```python
from build123d import *

# Parameters (mm, degrees)
F0_W     = 32
F0_H     = 36.5
F0_W_2   = 28
F0_H_2   = 32.5
F1_DEPTH = 9
F0_R     = 0.9
F2_DEPTH = 2
F3_DEPTH = 5
F4_W     = 28
F4_H     = 2
F5_DEPTH = 2
F6_W     = 20
F6_H     = 7
F7_DEPTH = 2
F8_W     = 29
F8_H     = 27.5
F9_DEPTH = 5
F11_D    = 2.4
F13_D    = 2.4


with BuildPart() as f1:
    # F0 (on Top) → F1 (new body)
    with BuildSketch(Plane.XY):
        with Locations((-98.1993639427, 45.2269401511)):
            Rectangle(F0_W, F0_H)
        with Locations((-98.1993639427, 45.2269401511)):
            Rectangle(F0_W_2, F0_H_2, mode=Mode.SUBTRACT)
    extrude(amount=F1_DEPTH)

    # F0 (on Top) → F2 (join)
    with BuildSketch(Plane.XY):
        with Locations((-98.1993639427, 45.2269401511)):
            Rectangle(F0_W_2, F0_H_2)
        with Locations((-108.1993639427, 32.9769401511)):
            Circle(F0_R, mode=Mode.SUBTRACT)
        with Locations((-88.1993639427, 32.9769401511)):
            Circle(F0_R, mode=Mode.SUBTRACT)
        with Locations((-108.1993639427, 45.4769401511)):
            Circle(F0_R, mode=Mode.SUBTRACT)
        with Locations((-88.1993639427, 45.4769401511)):
            Circle(F0_R, mode=Mode.SUBTRACT)
    extrude(amount=F2_DEPTH)

    # F0 (on Top) → F3 (join)
    with BuildSketch(Plane.XY):
        with Locations((-108.1993639427, 32.9769401511)):
            Circle(F0_R)
        with Locations((-108.1993639427, 45.4769401511)):
            Circle(F0_R)
        with Locations((-88.1993639427, 32.9769401511)):
            Circle(F0_R)
        with Locations((-88.1993639427, 45.4769401511)):
            Circle(F0_R)
    extrude(amount=F3_DEPTH)

    # F4 (on face) → F5 (cut, through all)
    with BuildSketch(Plane.XZ.offset(-26.9769401511)):
        with Locations((-98.1993639427, 6)):
            Rectangle(F4_W, F4_H)
    extrude(amount=-F5_DEPTH, mode=Mode.SUBTRACT)

    # F6 (on face) → F7 (cut, through all)
    with BuildSketch(Plane(origin=(0, 63.4769401511, 0), x_dir=(-1, 0, 0), z_dir=(0, 1, 0))):
        with Locations((98.1993639427, 5.5)):
            Rectangle(F6_W, F6_H)
    extrude(amount=-F7_DEPTH, mode=Mode.SUBTRACT)

    # F8 (on face) → F9 (join)
    with BuildSketch(Plane(origin=(0, 0, 0), x_dir=(1, 0, 0), z_dir=(0, 0, -1))):
        with Locations((-98.1993639427, -46.4769401511)):
            Rectangle(F8_W, F8_H)
        with BuildLine():
            ThreePointArc((-99.1993639427, -35.7269401511), (-98.1993639427, -34.7269401511), (-97.1993639427, -35.7269401511))
            Line((-97.1993639427, -35.7269401511), (-86.6993639427, -35.7269401511))
            Line((-86.6993639427, -35.7269401511), (-86.6993639427, -45.4769401511))
            ThreePointArc((-86.6993639427, -45.4769401511), (-85.9922571615, -45.7698333699), (-85.6993639427, -46.4769401511))
            ThreePointArc((-85.6993639427, -46.4769401511), (-85.9922571615, -47.1840469322), (-86.6993639427, -47.4769401511))
            Line((-86.6993639427, -47.4769401511), (-86.6993639427, -57.2269401511))
            Line((-86.6993639427, -57.2269401511), (-97.1993639427, -57.2269401511))
            ThreePointArc((-97.1993639427, -57.2269401511), (-98.1993639427, -58.2269401511), (-99.1993639427, -57.2269401511))
            Line((-99.1993639427, -57.2269401511), (-109.6993639427, -57.2269401511))
            Line((-109.6993639427, -57.2269401511), (-109.6993639427, -47.4769401511))
            ThreePointArc((-109.6993639427, -47.4769401511), (-110.6993639427, -46.4769401511), (-109.6993639427, -45.4769401511))
            Line((-109.6993639427, -45.4769401511), (-109.6993639427, -35.7269401511))
            Line((-109.6993639427, -35.7269401511), (-99.1993639427, -35.7269401511))
        make_face(mode=Mode.SUBTRACT)
        with BuildLine():
            Line((-86.6993639427, -47.4769401511), (-86.6993639427, -45.4769401511))
            ThreePointArc((-86.6993639427, -45.4769401511), (-87.6993639427, -46.4769401511), (-86.6993639427, -47.4769401511))
        make_face()
        with BuildLine():
            ThreePointArc((-85.6993639427, -46.4769401511), (-85.9922571615, -45.7698333699), (-86.6993639427, -45.4769401511))
            Line((-86.6993639427, -45.4769401511), (-86.6993639427, -47.4769401511))
            ThreePointArc((-86.6993639427, -47.4769401511), (-85.9922571615, -47.1840469322), (-85.6993639427, -46.4769401511))
        make_face()
        with BuildLine():
            Line((-99.1993639427, -35.7269401511), (-97.1993639427, -35.7269401511))
            ThreePointArc((-97.1993639427, -35.7269401511), (-98.1993639427, -34.7269401511), (-99.1993639427, -35.7269401511))
        make_face()
        with BuildLine():
            ThreePointArc((-99.1993639427, -35.7269401511), (-98.1993639427, -36.7269401511), (-97.1993639427, -35.7269401511))
            Line((-97.1993639427, -35.7269401511), (-99.1993639427, -35.7269401511))
        make_face()
        with BuildLine():
            ThreePointArc((-108.6993639427, -46.4769401511), (-108.9922571615, -45.7698333699), (-109.6993639427, -45.4769401511))
            Line((-109.6993639427, -45.4769401511), (-109.6993639427, -47.4769401511))
            ThreePointArc((-109.6993639427, -47.4769401511), (-108.9922571615, -47.1840469322), (-108.6993639427, -46.4769401511))
        make_face()
        with BuildLine():
            Line((-109.6993639427, -47.4769401511), (-109.6993639427, -45.4769401511))
            ThreePointArc((-109.6993639427, -45.4769401511), (-110.6993639427, -46.4769401511), (-109.6993639427, -47.4769401511))
        make_face()
        with BuildLine():
            Line((-99.1993639427, -57.2269401511), (-97.1993639427, -57.2269401511))
            ThreePointArc((-97.1993639427, -57.2269401511), (-98.1993639427, -56.2269401511), (-99.1993639427, -57.2269401511))
        make_face()
        with BuildLine():
            ThreePointArc((-99.1993639427, -57.2269401511), (-98.1993639427, -58.2269401511), (-97.1993639427, -57.2269401511))
            Line((-97.1993639427, -57.2269401511), (-99.1993639427, -57.2269401511))
        make_face()
    extrude(amount=F9_DEPTH)

    # F11 (through all)
    with Locations(Plane(origin=(0, 60.2269401511, 0), x_dir=(-1, 0, 0), z_dir=(0, 1, 0))):
        with Locations((98.1993639427, -2.5)):
            Hole(F11_D / 2)

    # F13 (through all)
    with Locations(Plane(origin=(-112.6993639427, 0, 0), x_dir=(0, -1, 0), z_dir=(-1, 0, 0))):
        with Locations((-46.4769401511, -2.5)):
            Hole(F13_D / 2)


solid = f1.part
```
The listing builds one solid part. Answer for the finished solid, in the listing's coordinates (mm). A direction names the side the tool comes from. Coordinates: 2 decimals unless noted, no trailing zeros. Loops run counter-clockwise (first coordinate to the right, second up) from the corner with the lowest first, then second, coordinate; pieces in that order, holes last. Notation, with made-up numbers: (57.25, -22) - (67.25, -22) arc R30 cw to (67.25, 17) - close; hole circle Ø10 at (64.5, -7). An arc over 180 degrees is marked (long way). Use a Markdown table: item, result. Add a question column.
1) Find the intervals of material crossed by line 1 (X direction, y = 55, z = 5.75); line 2 (Y direction, x = -95.5, z = -2.5); line 3 (X direction, y = 34.85, z = -2.5), in increasing order.
2) For faces 3 (the cylindrical face through (-111.116, 46.217, -3.671)), 4 (the flat face through (-108, 33, 5)), 5 (the flat face through (-98, 28, 5)), 6 (the cylindrical face through (-98.177, 56.227, -4.273)), 7 (the flat face through (-86, 61.477, 5)), determine the directions among +Z, -Z, +X, -X, +Y, -Y from which every point of the face is accessible in a straight line to the end or side of a thin tool.
3) The part is cut by section D-D, the plane z = -0.5. Give the vertices of the cut face in (x, y).
4) The part is cut by section A-A, the plane x = -95. Give the vertices of the cut face in (y, z).
5) The part is cut by section C-C, the plane z = -2.5. Give the vertices of the cut face in (x, y), and give its area (3 significant figures).
6) The mould has two halves that part along X. Classify faces 1 (the cylindrical face through (-98.221, 36.727, -4.273)), 2 (the flat face through (-98, 60.227, -1)): released by +X, released by -X, zero draft, split by the parting line, or undercut.
7) Given pin 1 (2.5 mm diameter, centred on y = 51, z = -1.5, fed in from -X); pin 2 (17 mm diameter, centred on x = -102.5, y = 42.5, fed in from -Z); pin 3 (2 mm diameter, centred on x = -94.5, y = 53.5, fed in from +Z); pin 4 (2.5 mm diameter, centred on x = -105.5, z = -2.5, fed in from +Y), each flat-ended and moving along its own axis, determine where each tip first touches the part or whether it passes through.
8) The part is cut by section B-B, the plane y = 35. Give the vertices of the cut face in (x, z).
Here are the results:
| question | item | result |
|---|---|---|
| 1 | line 1 | x = -114.2 to -112.2, -84.2 to -82.2 |
| 1 | line 2 | y = 32.73 to 35.73, 57.23 to 60.23 |
| 1 | line 3 | x = -112.7 to -99.4, -97 to -83.7 |
| 2 | face 3 | +X, -X |
| 2 | face 4 | +Z, -Y |
| 2 | face 5 | -Y |
| 2 | face 6 | -Z |
| 2 | face 7 | +Z |
| 3 | outline | (-112.7, 32.73) - (-83.7, 32.73) - (-83.7, 60.23) - (-112.7, 60.23) - close; hole (-109.7, 35.73) - (-99.2, 35.73) arc R1 cw to (-97.2, 35.73) - (-86.7, 35.73) - (-86.7, 45.48) arc R1 cw to (-86.7, 47.48) - (-86.7, 57.23) - (-97.2, 57.23) arc R1 cw to (-99.2, 57.23) - (-109.7, 57.23) - (-109.7, 47.48) arc R1 cw to (-109.7, 45.48) - close |
| 4 | outline | (26.98, 0) - (32.73, 0) - (32.73, -5) - (35.73, -5) - (35.73, 0) - (57.23, 0) - (57.23, -5) - (60.23, -5) - (60.23, 0) - (63.48, 0) - (63.48, 2) - (28.98, 2) - (28.98, 5) - (26.98, 5) - close; (26.98, 7) - (28.98, 7) - (28.98, 9) - (26.98, 9) - close |
| 5 | outline | (-112.7, 32.73) - (-99.4, 32.73) - (-99.4, 35.73) - (-109.7, 35.73) - (-109.7, 45.28) - (-112.7, 45.28) - close; (-112.7, 47.68) - (-109.7, 47.68) - (-109.7, 57.23) - (-99.4, 57.23) - (-99.4, 60.23) - (-112.7, 60.23) - close; (-97, 32.73) - (-83.7, 32.73) - (-83.7, 45.28) - (-86.7, 45.28) - (-86.7, 35.73) - (-97, 35.73) - close; (-97, 57.23) - (-86.7, 57.23) - (-86.7, 47.68) - (-83.7, 47.68) - (-83.7, 60.23) - (-97, 60.23) - close |
| 5 | area | 274 mm^2 |
| 6 | face 1 | undercut |
| 6 | face 2 | zero draft |
| 7 | pin 1 | stops at x = -112.7 |
| 7 | pin 2 | stops at z = -5 |
| 7 | pin 3 | stops at z = 2 |
| 7 | pin 4 | stops at y = 60.23 |
| 8 | outline | (-114.2, 0) - (-112.7, 0) - (-112.7, -5) - (-83.7, -5) - (-83.7, 0) - (-82.2, 0) - (-82.2, 9) - (-84.2, 9) - (-84.2, 2) - (-112.2, 2) - (-112.2, 9) - (-114.2, 9) - close; hole circle Ø2.4 at (-98.2, -2.5) |
